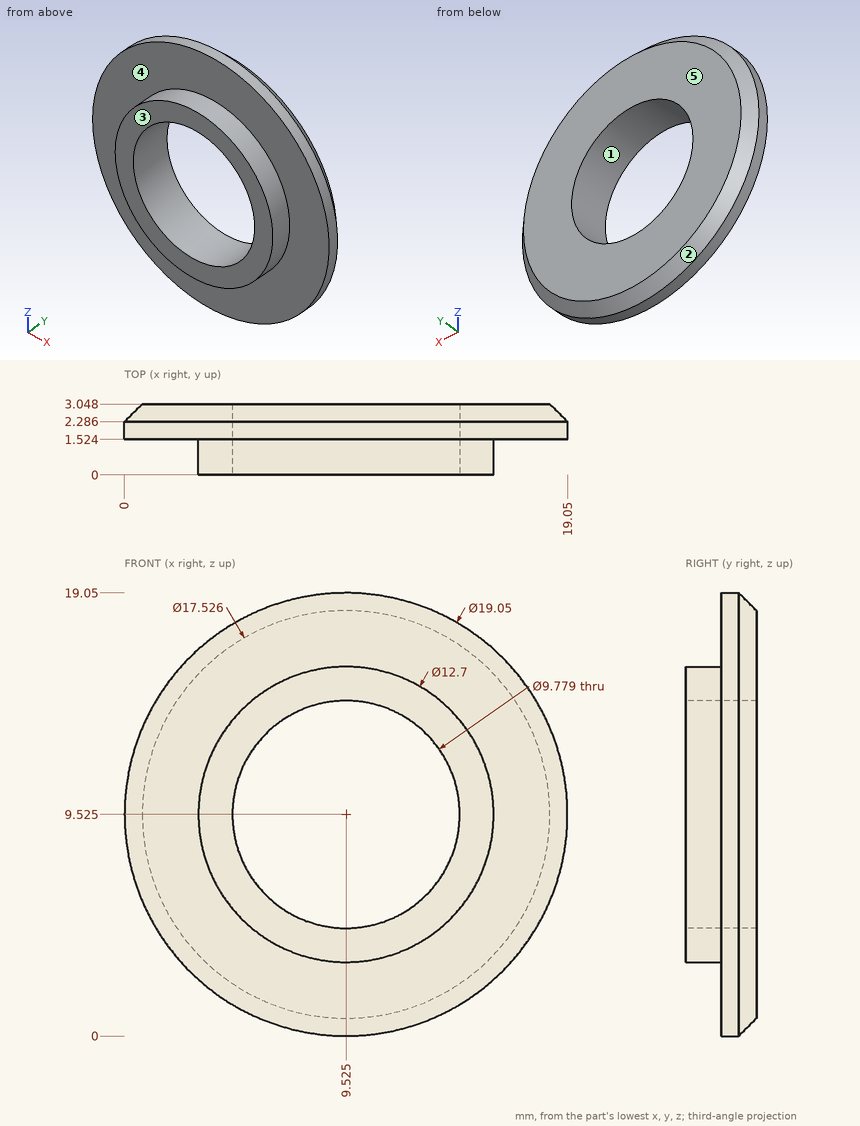
Could you check a few things on this drawing? It's one solid part, dimensions in mm from its lowest x, y, z. A direction names the side the tool comes from. Round coordinates to 2 decimals unless told otherwise and drop trailing zeros.
Q1. Which directions (+Z, -Z, +X, -X, +Y, -Y) give clear straight access to the entire face, cutting with the end or side of a thin tool? Please do the marked faces 4 and 5.
Q2. Will these pins go through, and if not, where does the flat tip stop? P1, Ø1.5, axis at y = 2.5, z = 15, coming from the -X side; P2, Ø1, axis at x = 6, z = 11, coming from the +Y side; P3, Ø1.5, axis at x = 12.5, y = 2, coming from the -Z side.
Q3. Please list where these lines run through material, in increasing order: probe 1 along X at (y, z) = (1.15, 9.5); probe 2 along X at (y, z) = (1.7, 9.5); probe 3 along Y at (x, z) = (16, 12).
Q4. If we mould it in two halves opening along X, with no side actions, what happens to the marked faces 1, 2 and 3? For each: +X half, -X half, draft (parallel to the pull), parting line (faces both ways), or undercut.
Answer below:
1. face 4: -Y
1. face 5: +Z, -Z, +X, -X, +Y
2. P1: stops at x = 1.27
2. P2: passes through
2. P3: stops at z = 0.26
3. probe 1: x = 3.18 to 4.64, 14.41 to 15.87
3. probe 2: x = 0 to 4.64, 14.41 to 19.05
3. probe 3: y = 1.52 to 3.05
4. face 1: undercut
4. face 2: parting line
4. face 3: draft
